Drawing for the job (mm, zero at the part's lowest x, y, z). A direction names the side the tool comes from. Round coordinates to 2 decimals unless told otherwise and drop trailing zeros. Loops run counter-clockwise (first coordinate to the right, second up) from the corner with the lowest first, then second, coordinate; pieces in that order, holes last. Notation, with made-up numbers: M -9.75,10.25 L 31.25,10.25 A19 cw 31.25,22.25 Z; hole C 66.5,-16 d8. An arc over 180 degrees is marked long. Write each question's results on one line, items separated by ' | '.
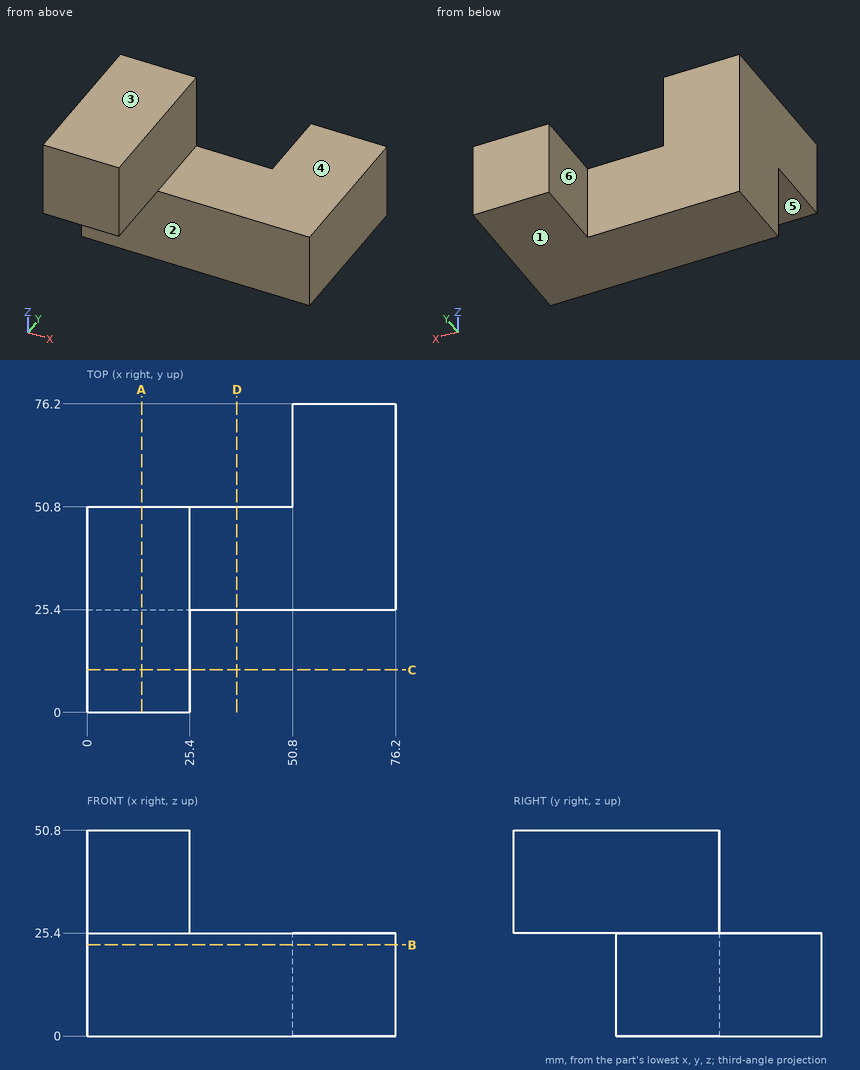
Item 1: Wall check: L1, parallel to X at y = 25.5, z = 30; L2, parallel to Y at x = 8, z = 6.5. Give the ranges that are in metal, low to high.
Filled sheet:
L1: 0 to 25.4 | L2: 25.4 to 50.8
Item 2: Band-saw the part on A-A on x = 13.5. Give the cut face in (y, z).
Filled sheet:
outline: M 0,25.4 L 25.4,25.4 L 25.4,0 L 50.8,0 L 50.8,50.8 L 0,50.8 Z
Item 3: Two-plate mould, pull along Z, no slides. Class the marked faces 1, 2 and 3: +Z half, -Z half, draft (parallel to the pull), parting line (faces both ways), or undercut.
Filled sheet:
face 1: -Z half | face 2: draft | face 3: +Z half
Item 4: Drop flat-ended pins along their axis: P1, Ø12, axis at x = 66.5, z = 11.5, coming from the -Y side; P2, Ø3, axis at x = 42.5, y = 42, coming from the +Z side; P3, Ø12.5, axis at y = 35.5, z = 36.5, coming from the +X side. Give the stop position or say it passes through.
Filled sheet:
P1: y = 25.4 | P2: z = 25.4 | P3: x = 25.4
Item 5: Which spindle directions (+Z, -Z, +X, -X, +Y, -Y) get a long thin tool onto all of the face, cutting with end or side? Do the marked faces 4, 5 and 6. Say none if no direction does.
Filled sheet:
face 4: +Z, +X, +Y, -Y | face 5: -Z, +X, -X, -Y | face 6: +Z, -Z, -X, +Y
Item 6: Band-saw the part on C-C on y = 10.5. Give the cut face in (x, z), and give its area (3 significant figures).
Filled sheet:
outline: M 0,25.4 L 25.4,25.4 L 25.4,50.8 L 0,50.8 Z | area: 645 mm^2
Item 7: Band-saw the part on B-B on z = 22.5. Give the cut face in (x, y).
Filled sheet:
outline: M 0,25.4 L 76.2,25.4 L 76.2,76.2 L 50.8,76.2 L 50.8,50.8 L 0,50.8 Z
Item 8: Band-saw the part on D-D on x = 37. Give the cut face in (y, z), and give its area (3 significant figures).
Filled sheet:
outline: M 25.4,0 L 50.8,0 L 50.8,25.4 L 25.4,25.4 Z | area: 645 mm^2
